Part model, mm, in its own coordinate system. A direction names the side the tool comes from. Round coordinates to 2 decimals unless told otherwise and drop trailing zeros. Loops run counter-clockwise (first coordinate to the right, second up) from the corner with the lowest first, then second, coordinate; pieces in that order, holes last.
1) Mould opens along Z. For faces 1 (the cylindrical face through (-80.12, 5.01, 66.12)), 2 (the cylindrical face through (13.738, 26.116, -5.116)) say: +Z half, -Z half, draft (parallel to the pull), parting line (faces both ways), or undercut.
2) Probe line 1 (Z direction, x = -68, y = 42); line 2 (Z direction, x = 12.5, y = 24.5); line 3 (X direction, y = 7.5, z = 27). List the from-to ranges inside material, lowest first.
3) Band-saw the part on D-D, the plane y = 35. State how many separate pieces and enclosed holes the cut face has, then the cut area to 3 significant figures.
4) Band-saw the part on A-A, the plane z = 24. Write the cut outline in (x, y), then the cut area to 3 significant figures.
5) Band-saw the part on C-C, the plane y = 52. Write the cut outline in (x, z), then the cut area to 3 significant figures.
6) Band-saw the part on B-B, the plane x = -55. Write the cut outline in (y, z), then the cut area to 3 significant figures.
7) 3-axis set-ups, long thin cutter, end or side, ignore diameter. For faces 3 (the flat face through (-57.4, 27.9, -2.54)), 4 (the flat face through (27.581, 5, 31)), 5 (the flat face through (-75.333, 19, 61)): which of +Z, -Z, +X, -X, +Y, -Y reach the whole face in a straight line?
8) Drop flat-ended pins along their axis: P1, Ø3, axis at x = 14.5, y = 27.58, coming from the +Z side; P2, Ø12, axis at y = 20, z = 59.5, coming from the +X side; P3, Ø4.5, axis at y = 19.5, z = 64.5, coming from the -X side; P4, Ø4.5, axis at x = 38.76, z = 3.56, coming from the +Y side. Give the stop position or say it passes through.
from build123d import *

# Parameters (mm, degrees)
SKETCH2_R                 = 22.50059
BOSS_EXTRUDE1_DEPTH       = 7.62
SKETCH6_R                 = 22.50059
SKETCH6_R_2               = 9.144
BOSS_EXTRUDE2_DEPTH       = 5.08
SKETCH7_R                 = 1.651
CUT_EXTRUDE1_DEPTH        = 7.62
SKETCH8_R                 = 1.651
CUT_EXTRUDE2_DEPTH        = 107.53344751
TAP_DRILL_FOR_6_32_TAP1_D = 2.7051
SKETCH11_W                = 15.24
SKETCH11_H                = 10.16
BOSS_EXTRUDE3_DEPTH       = 23.08987
TAP_DRILL_FOR_6_32_TAP2_D = 2.7051


with BuildPart() as part:
    # Sketch2 → Boss-Extrude1 (new, symmetric)
    with BuildSketch(Plane.XY):
        with BuildLine():
            Line((-47.752, 55.16118), (0, 55.16118))
            ThreePointArc((0, 55.16118), (19.502422218, 47.083012218), (27.58059, 27.58059))
            Line((27.58059, 27.58059), (27.58059, 10.16))
            Line((27.58059, 10.16), (42.82059, 10.16))
            Line((42.82059, 10.16), (42.82059, 0))
            Line((42.82059, 0), (-42.82059, 0))
            Line((-42.82059, 0), (-90.57259, 0))
            Line((-90.57259, 0), (-90.57259, 10.16))
            Line((-90.57259, 10.16), (-75.33259, 10.16))
            Line((-75.33259, 10.16), (-75.33259, 27.58059))
            ThreePointArc((-75.33259, 27.58059), (-67.254422218, 47.083012218), (-47.752, 55.16118))
        make_face()
        with Locations((0, 27.58059)):
            Circle(SKETCH2_R, mode=Mode.SUBTRACT)
        with Locations((-47.752, 27.58059)):
            Circle(SKETCH2_R, mode=Mode.SUBTRACT)
    extrude(amount=BOSS_EXTRUDE1_DEPTH, both=True)

    # Sketch6 → Boss-Extrude2 (add)
    # profile 1 of 2: a face of its own
    with BuildSketch(Plane(origin=(0, 0, -7.62), x_dir=(-1, 0, 0), z_dir=(0, 0, -1))):
        with Locations((0, 27.58059)):
            Circle(SKETCH6_R)
        with Locations((0, 27.58059)):
            Circle(SKETCH6_R_2, mode=Mode.SUBTRACT)
    # profile 2 of 2: a face of its own
    with BuildSketch(Plane(origin=(0, 0, -7.62), x_dir=(-1, 0, 0), z_dir=(0, 0, -1))):
        with Locations((47.752, 27.58059)):
            Circle(SKETCH6_R)
        with Locations((47.752, 27.58059)):
            Circle(SKETCH6_R_2, mode=Mode.SUBTRACT)
    extrude(amount=-BOSS_EXTRUDE2_DEPTH)

    # Sketch7 → Cut-Extrude1 (cut)
    with BuildSketch(Plane(origin=(0, 0, -7.62), x_dir=(-1, 0, 0), z_dir=(0, 0, -1))):
        with Locations((-14.49959, 27.58059)):
            Circle(SKETCH7_R)
        with Locations((14.49959, 27.58059)):
            Circle(SKETCH7_R)
    extrude(amount=-CUT_EXTRUDE1_DEPTH, mode=Mode.SUBTRACT)

    # Sketch8 → Cut-Extrude2 (cut, through all)
    with BuildSketch(Plane.XY.offset(-2.54)):
        with Locations((-33.25241, 27.58059)):
            Circle(SKETCH8_R)
        with Locations((-62.25159, 27.58059)):
            Circle(SKETCH8_R)
    extrude(amount=-CUT_EXTRUDE2_DEPTH, mode=Mode.SUBTRACT)

    # Tap Drill for #6-32 Tap1 (through all)
    with Locations(Plane(origin=(0, 10.16, 0), x_dir=(1, 0, 0), z_dir=(0, 1, 0))):
        with Locations((-79.39659, 3.556), (-86.50859, -3.556)):
            tap_drill_for_6_32_tap1 = Hole(TAP_DRILL_FOR_6_32_TAP1_D / 2)

    # Mirror1: Tap Drill for #6-32 Tap1 across plane
    add(tap_drill_for_6_32_tap1.mirror(Plane.ZY.offset(23.876)), mode=Mode.SUBTRACT)

    # Sketch11 → Boss-Extrude3 (add)
    with BuildSketch(Plane.XY.offset(7.62)):
        with Locations((-82.95259, 5.08)):
            Rectangle(SKETCH11_W, SKETCH11_H)
        with Locations((35.20059, 5.08)):
            Rectangle(SKETCH11_W, SKETCH11_H)
    extrude(amount=BOSS_EXTRUDE3_DEPTH)

    # Mirror5: part across plane


with BuildPart() as part_1:
    add(part.part)
    add(part.part.mirror(Plane.XY.offset(30.70987)))

    # Tap Drill for #6-32 Tap2 (through all)
    with Locations(Plane(origin=(0, 10.16, 0), x_dir=(1, 0, 0), z_dir=(0, 1, 0))):
        with Locations((-82.95259, -30.70987), (-82.95259, -45.94987), (-82.95259, -15.46987)):
            tap_drill_for_6_32_tap2 = Hole(TAP_DRILL_FOR_6_32_TAP2_D / 2)

    # Mirror6: Tap Drill for #6-32 Tap2 across plane
    add(tap_drill_for_6_32_tap2.mirror(Plane.ZY.offset(23.876)), mode=Mode.SUBTRACT)


solid = part_1.part
Reported:
1. face 1: undercut
1. face 2: draft
2. line 1: z = -7.62 to 7.62, 53.8 to 69.04
2. line 2: z = -7.62 to -2.54, 63.96 to 69.04
2. line 3: x = -90.57 to -75.33, 27.58 to 42.82
3. separate pieces: 6
3. enclosed holes: 0
3. area: 1,130 mm2
4. outline: (-90.57, 0) - (-75.33, 0) - (-75.33, 10.16) - (-90.57, 10.16) - close; (27.58, 0) - (42.82, 0) - (42.82, 10.16) - (27.58, 10.16) - close
4. area: 310 mm2
5. outline: (-60.57, -7.62) - (12.82, -7.62) - (12.82, 7.62) - (-60.57, 7.62) - close; (-60.57, 53.8) - (12.82, 53.8) - (12.82, 69.04) - (-60.57, 69.04) - close
5. area: 2,240 mm2
6. outline: (0, -7.62) - (22.01, -7.62) - (22.01, -2.54) - (6.28, -2.54) - (6.28, 7.62) - (0, 7.62) - close; (0, 53.8) - (6.28, 53.8) - (6.28, 63.96) - (22.01, 63.96) - (22.01, 69.04) - (0, 69.04) - close; (33.16, -7.62) - (54.19, -7.62) - (54.19, 7.62) - (48.88, 7.62) - (48.88, -2.54) - (33.16, -2.54) - close; (33.16, 63.96) - (48.88, 63.96) - (48.88, 53.8) - (54.19, 53.8) - (54.19, 69.04) - (33.16, 69.04) - close
6. area: 673 mm2
7. face 3: none
7. face 4: +Y, -Y
7. face 5: +Z, -Z, -X, +Y
8. P1: passes through
8. P2: stops at x = 27.58
8. P3: stops at x = -75.33
8. P4: stops at y = 10.16
